Here's how the part is built. I have some questions about the finished solid (model axes, mm). Coordinates: 2 decimals unless noted, no trailing zeros. Write each loop counter-clockwise with the first axis right and the second up, starting at its lowest first coordinate (ties: lowest second). Pieces come first, ordered by that corner, then holes.
Item 1: If we section it at B-B (x = -168): Please give me the cut outline in (y, z).
Item 2: I'm going to push flat-ended pins straight in: pin 1 Ø1.5 at (x, y) = (-180.45, -4.75) entering from -Z; pin 2 Ø1.5 at (y, z) = (11, 1.5) entering from +X; pin 3 Ø1.5 at (y, z) = (-10.5, 1.5) entering from +X. Where does each tip first touch, or does it pass through?
Item 3: If we section it at A-A (y = 0): Please give me the cut outline in (x, z), then the cut area to 3 significant figures.
Item 4: If I drill on line 1 (X direction, y = -0.5, z = 2.3); line 2 (X direction, y = -5.5, z = 1.9); line 3 (X direction, y = 18, z = 3.75), over which ranges is the centre line in solid material (lowest first)?
Item 5: We'd pull the mould along X, two halves only. Please class faces 1 (the face through (-171, -10, 4)), 2 (the face through (-171.14, 15.12, 2.03)), 3 (the face through (-144.08, 8.75, 1.97)): +X half, -X half, draft (parallel to the pull), parting line (faces both ways), or undercut.
Item 6: If we section it at C-C (z = 1.45): Please give me the cut outline in (x, y), then the cut area to 3 significant figures.
Item 7: If we section it at D-D (x = -178.5): Please give me the cut outline in (y, z).
Autodesk Inventor part; units mm, degrees
ref_plane "Work Plane1" through (0, 0, 0) normal (0, 0, 1) x (1, 0, 0)
ref_plane "Work Plane2" through (0, 0, 0) normal (0, 0, 1) x (1, 0, 0)
ref_plane "YZ Plane" through (0, 0, 0) normal (1, 0, 0) x (0, 1, 0)
ref_plane "Work Plane1" through (0, 0, 0) normal (0, 0, 1) x (1, 0, 0)
ref_plane "Work Plane2" through (0, 0, 0) normal (0, 0, 1) x (1, 0, 0)
sketch "Sketch2" plane through (0, 0, 0) normal (0, 0, 1) x (1, 0, 0)
  circle A0 centre (-137.1735, 0) radius 1.55
  circle A1 centre (-165.1735, -28) radius 1.55
  circle A2 centre (-165.1735, 28) radius 1.55
  circle A3 centre (-184.9724, -19.799) radius 1.55
  circle A4 centre (-145.3745, 19.799) radius 1.55
  circle A5 centre (-145.3745, -19.799) radius 1.55
  circle A6 centre (-184.9724, 19.799) radius 1.55
  circle A7 centre (-193.1735, 0) radius 1.55
  circle A8 centre (-165.1735, 0) radius 32.5
  circle A9 centre (-165.1735, 0) radius 22.8355
  circle A10 centre (-165.1735, 0) radius 11
  arc A11 (-152.3597, 3.5298) -> (-152.6156, 4.3532) centre (-149.894, 4.7473) ccw
  arc A12 (-152.6156, 4.3532) -> (-168.7032, 12.8137) centre (-165.1735, 0) ccw
  arc A13 (-168.7032, 12.8137) -> (-169.5266, 12.5579) centre (-169.9208, 15.2795) ccw
  arc A14 (-169.5266, 12.5579) -> (-177.9872, -3.5298) centre (-165.1735, 0) ccw
  arc A15 (-177.9872, -3.5298) -> (-177.7313, -4.3532) centre (-180.4529, -4.7473) ccw
  arc A16 (-177.7313, -4.3532) -> (-161.6437, -12.8137) centre (-165.1735, 0) ccw
  arc A17 (-161.6437, -12.8137) -> (-160.8203, -12.5579) centre (-160.4261, -15.2795) ccw
  arc A18 (-160.8203, -12.5579) -> (-152.3597, 3.5298) centre (-165.1735, 0) ccw
  circle A19 centre (-165.1735, 0) radius 20.2623
  circle A20 centre (-169.9208, 15.2795) radius 1.55
  circle A21 centre (-160.4261, -15.2795) radius 1.55
  circle A22 centre (-180.4529, -4.7473) radius 1.55
  circle A23 centre (-149.894, 4.7473) radius 1.55
  circle A24 centre (-165.1735, 0) radius 13.291
  point P0 (0, 0)
extrude "Extrusion2" add sketch "Sketch2" along normal blind 4 contours A9 | A24 A11 | A18 A24 A16 A14 A12 | A24 A13 | A17 A24 | A24 A15 | A19 | A20 | A21 | A22 | A23
sketch "Sketch3" plane through (-165.1735, 0, 0) normal (0, 0, -1) x (-1, 0, 0)
  point P0 (-165.1735, 0)
  point P1 (-15.2795, 4.7473)
  point P2 (4.7473, 15.2795)
  point P3 (15.2795, -4.7473)
  point P4 (-4.7473, -15.2795)
hole "Hole1" at (-149.894, 4.7473, 0) at (-169.9208, 15.2795, 0) at (-180.4529, -4.7473, 0) at (-160.4261, -15.2795, 0) direction (0, 0, 1) diameter 2.459 end through all
properties part number "lagerblokje" material "Aluminum 6061"
Answer list:
1. outline: (-22.66, 0) - (-10.63, 0) - (-10.63, 4) - (-22.66, 4) - close; (10.63, 0) - (22.66, 0) - (22.66, 4) - (10.63, 4) - close
2. pin 1: passes through
2. pin 2: stops at x = -144.77
2. pin 3: stops at x = -144.52
3. outline: (-188.01, 0) - (-176.17, 0) - (-176.17, 4) - (-188.01, 4) - close; (-154.17, 0) - (-142.34, 0) - (-142.34, 4) - (-154.17, 4) - close
3. area: 94.7 mm2
4. line 1: x = -188 to -176.16, -154.18 to -142.34
4. line 2: x = -187.34 to -181.43, -179.48 to -174.7, -155.65 to -143.01
4. line 3: x = -179.23 to -151.12
5. face 1: draft
5. face 2: undercut
5. face 3: parting line
6. outline: circle Ø45.67 at (-165.17, 0); hole circle Ø2.46 at (-180.45, -4.75); hole circle Ø22 at (-165.17, 0); hole circle Ø2.46 at (-169.92, 15.28); hole circle Ø2.46 at (-160.43, -15.28); hole circle Ø2.46 at (-149.89, 4.75)
6. area: 1,240 mm2
7. outline: (-18.54, 0) - (18.54, 0) - (18.54, 4) - (-18.54, 4) - close
